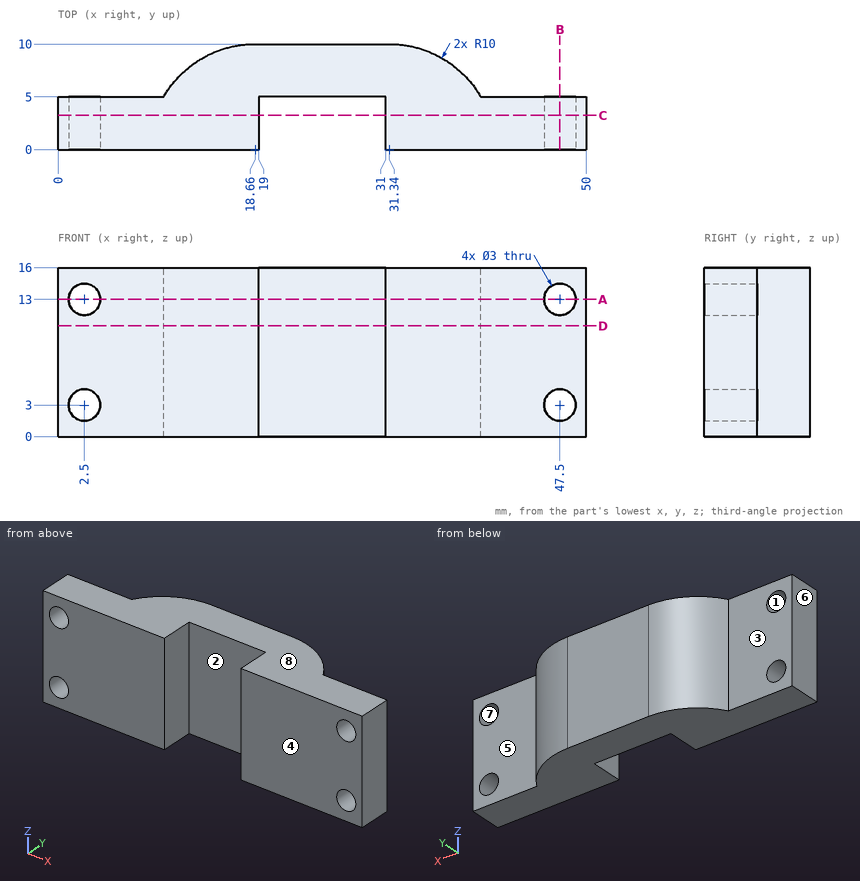
Can you work these out from the drawing? Everything is in mm from the part's minimum corner. A direction names the side the tool comes from. Give positions to 0.01 mm unless a question says otherwise; leave off trailing zeros. Loops run counter-clockwise (first coordinate to the right, second up) from the corner with the lowest first, then second, coordinate; pieces in that order, holes last. Notation, with made-up numbers: (-16, 67.5) -> (-10, 67.5) arc R19 ccw to (-10, 84.5) -> close; hole circle Ø10 at (-34.75, -21). An arc over 180 degrees is marked (long way). Return JSON: item names as keys, results as strings.
Item 1: I'm going to push flat-ended pins straight in: pin 1 (5 mm diameter, centred on y = 6, z = 3, fed in from -X); pin 2 (1 mm diameter, centred on x = 13.5, z = 12, fed in from +Y); pin 3 (4 mm diameter, centred on x = 2.5, z = 3, fed in from +Y); pin 4 (6 mm diameter, centred on x = 24, z = 3, fed in from -Y). Where does each tip first touch, or does it pass through?
Geometry results:
{"pin 1": "stops at x = 0", "pin 2": "stops at y = 8.85", "pin 3": "stops at y = 5", "pin 4": "stops at y = 5"}
Item 2: If we section it at A-A on z = 13: List the corners of the cut face in (x, y) for me.
Geometry results:
{"outline": "(0, 0) -> (1, 0) -> (1, 5) -> (0, 5) -> close; (4, 0) -> (19, 0) -> (19, 5) -> (31, 5) -> (31, 0) -> (46, 0) -> (46, 5) -> (40, 5) arc R10 ccw to (31.34, 10) -> (18.66, 10) arc R10 ccw to (10, 5) -> (4, 5) -> close; (49, 0) -> (50, 0) -> (50, 5) -> (49, 5) -> close"}
Item 3: If we section it at D-D on z = 10.5: List the corners of the cut face in (x, y) for me.
Geometry results:
{"outline": "(0, 0) -> (19, 0) -> (19, 5) -> (31, 5) -> (31, 0) -> (50, 0) -> (50, 5) -> (40, 5) arc R10 ccw to (31.34, 10) -> (18.66, 10) arc R10 ccw to (10, 5) -> (0, 5) -> close"}
Item 4: We'd pull the mould along Z, two halves only. Please class the marked faces 6, 7 and 8: +Z half, -Z half, draft (parallel to the pull), parting line (faces both ways), or undercut.
Geometry results:
{"face 6": "draft", "face 7": "undercut", "face 8": "+Z half"}
Item 5: Which directions (+Z, -Z, +X, -X, +Y, -Y) give clear straight access to the entire face, cutting with the end or side of a thin tool? Please do the marked faces 1, 2, 3, 4 and 5.
Geometry results:
{"face 1": "+Y, -Y", "face 2": "+Z, -Z, -Y", "face 3": "+Z, -Z, -X, +Y", "face 4": "+Z, -Z, +X, -X, -Y", "face 5": "+Z, -Z, +X, +Y"}
Item 6: If we section it at C-C on y = 3.25: List the corners of the cut face in (x, z) for me, plus the area to 3 significant figures.
Geometry results:
{"outline": "(0, 0) -> (19, 0) -> (19, 16) -> (0, 16) -> close; (31, 0) -> (50, 0) -> (50, 16) -> (31, 16) -> close; hole circle Ø3 at (2.5, 3); hole circle Ø3 at (2.5, 13); hole circle Ø3 at (47.5, 3); hole circle Ø3 at (47.5, 13)", "area": "580 mm²"}
Item 7: If we section it at B-B on x = 47.5: List the corners of the cut face in (y, z) for me, plus the area to 3 significant figures.
Geometry results:
{"outline": "(0, 0) -> (5, 0) -> (5, 1.5) -> (0, 1.5) -> close; (0, 4.5) -> (5, 4.5) -> (5, 11.5) -> (0, 11.5) -> close; (0, 14.5) -> (5, 14.5) -> (5, 16) -> (0, 16) -> close", "area": "50.0 mm²"}
Item 8: I need wall thicknesses on L1, parallel to X at y = 2.75, z = 3; L2, parallel to Z at x = 2.5, y = 2.85; L3, parallel to X at y = 1, z = 13.5 (1 decimal). Which ranges of each line are inside material? Lowest first, please. Write a range as from..to.
Geometry results:
{"L1": "x = 0..1, 4..19, 31..46, 49..50", "L2": "z = 0..1.5, 4.5..11.5, 14.5..16", "L3": "x = 0..1.1, 3.9..19, 31..46.1, 48.9..50"}
